Here's the drawing with two shaded views (mm, measured from the low corner). I have some questions. Round coordinates to 2 decimals unless told otherwise and drop trailing zeros. Write each loop counter-clockwise with the first axis right and the second up, starting at its lowest first coordinate (ties: lowest second). Pieces come first, ordered by that corner, then holes.
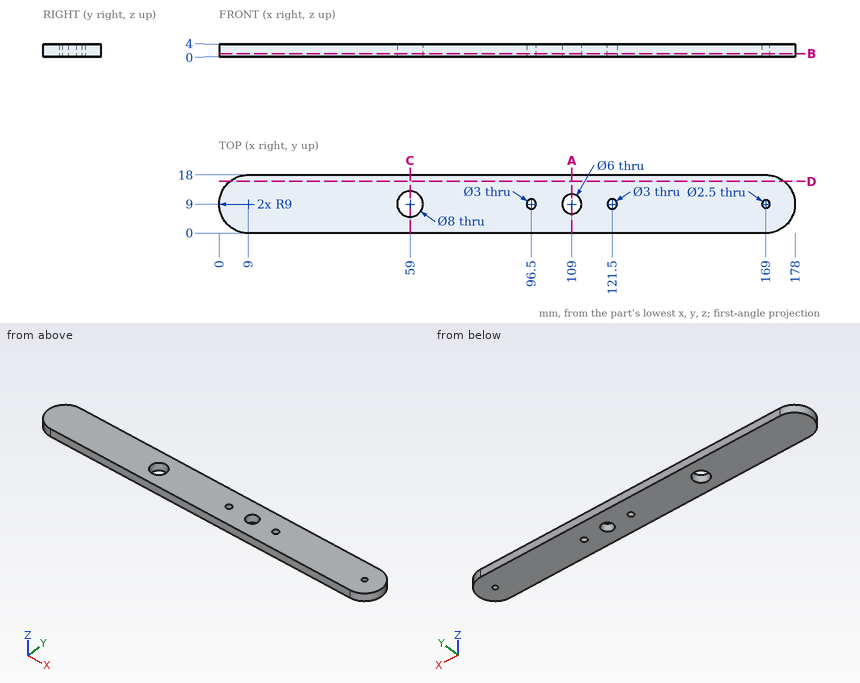
Q1. Imagine slicing it at B-B, the plane z = 1.05. Write out the boundary of the cut face in (x, y), then the cut area to 3 significant figures.
Q2. If I drill on L1, parallel to X at y = 10, z = 3.7; L2, parallel to X at y = 11.5, z = 2.2; L3, parallel to Y at x = 169, z = 1.6, over which ranges is the centre line in solid material (lowest first)?
Q3. Imagine slicing it at A-A, the plane x = 109. Write out the boundary of the cut face in (y, z), then the cut area to 3 significant figures.
Q4. Imagine slicing it at D-D, the plane y = 16. Write out the boundary of the cut face in (x, z).
Q5. Imagine slicing it at C-C, the plane x = 59. Write out the boundary of the cut face in (y, z), then the cut area to 3 significant figures.
Results found:
1. outline: (9, 0) - (169, 0) arc R9 ccw to (169, 18) - (9, 18) arc R9 ccw to start; hole circle Ø8 at (59, 9); hole circle Ø3 at (96.5, 9); hole circle Ø6 at (109, 9); hole circle Ø3 at (121.5, 9); hole circle Ø2.5 at (169, 9)
1. area: 3,040 mm2
2. L1: x = 0.06 to 55.13, 62.87 to 95.38, 97.62 to 106.17, 111.83 to 120.38, 122.62 to 168.25, 169.75 to 177.94
2. L2: x = 0.35 to 55.88, 62.12 to 107.34, 110.66 to 177.65
2. L3: y = 0 to 7.75, 10.25 to 18
3. outline: (0, 0) - (6, 0) - (6, 4) - (0, 4) - close; (12, 0) - (18, 0) - (18, 4) - (12, 4) - close
3. area: 48.0 mm2
4. outline: (3.34, 0) - (174.66, 0) - (174.66, 4) - (3.34, 4) - close
5. outline: (0, 0) - (5, 0) - (5, 4) - (0, 4) - close; (13, 0) - (18, 0) - (18, 4) - (13, 4) - close
5. area: 40.0 mm2
